Could you check a few things on this model? Use its own coordinates, in mm. Face numbers are marked on the shaded views. A direction names the side the tool comes from. Give positions to 0.01 mm unless a question says otherwise; leave off trailing zeros. Write each loop counter-clockwise with the first axis right and the second up, starting at its lowest first coordinate (ties: lowest second). Pieces come first, ordered by that corner, then holes. Notation, with made-up numbers: M 36.5,-11.75 L 59.5,-11.75 A15 cw 59.5,12.25 Z; hole C 49,-37 d3. An arc over 180 degrees is marked long. Answer as a JSON object with one key per item and string values. Group by question number.
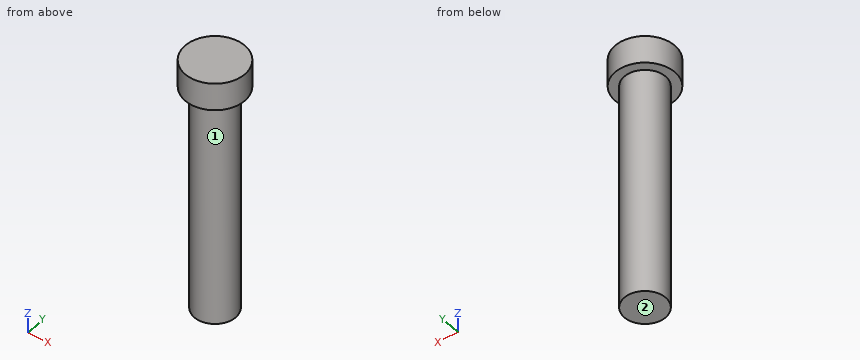
```python
from build123d import *

# Parameters (mm, degrees)
ESQUISSE1_R                    = 2.25
ESQUISSE1_R_2                  = 1.25
EXTRU_MINCE1_DEPTH             = 25
BOSS_EXTRU_1_REACH             = 14.899
ESQUISSE2_R                    = 1.25
BOSS_EXTRU_1_DIRECTION_2_REACH = 14.899
ESQUISSE3_R                    = 3.25
BOSS_EXTRU_2_DEPTH             = 3


with BuildPart() as part:
    # Esquisse1 → Extru.-Mince1 (new body)
    with BuildSketch(Plane.XY):
        Circle(ESQUISSE1_R)
        Circle(ESQUISSE1_R_2, mode=Mode.SUBTRACT)
    extrude(amount=EXTRU_MINCE1_DEPTH)

    # Boss.-Extru.1: up to this face of the body (flat: up to its plane)
    boss_extru_1_end = Plane(part.part.faces().sort_by_distance((-2.18636039, 0, 0))[0])
    # Esquisse2 → Boss.-Extru.1 (add, up to the picked face)
    with BuildSketch(Plane(origin=(0, 0, 12.5), x_dir=(-1, 0, 0), z_dir=(0, 0, -1)), mode=Mode.PRIVATE) as boss_extru_1_sk1:
        Circle(ESQUISSE2_R)
    boss_extru_1_tool1 = split(extrude(boss_extru_1_sk1.sketch, amount=BOSS_EXTRU_1_REACH, mode=Mode.PRIVATE), bisect_by=boss_extru_1_end, keep=Keep.BOTH, mode=Mode.PRIVATE)
    add(boss_extru_1_tool1.solids().sort_by(Axis((0, 0, 12.5), (0, 0, -1)))[0])

    # Boss.-Extru.1 direction 2: up to this face of the body (flat: up to its plane)
    boss_extru_1_direction_2_end = Plane(part.part.faces().sort_by_distance((-2.18636039, 0, 25))[0])
    # Esquisse2 → Boss.-Extru.1 direction 2 (add, up to the picked face)
    with BuildSketch(Plane(origin=(0, 0, 12.5), x_dir=(-1, 0, 0), z_dir=(0, 0, -1)), mode=Mode.PRIVATE) as boss_extru_1_direction_2_sk1:
        Circle(ESQUISSE2_R)
    boss_extru_1_direction_2_tool1 = split(extrude(boss_extru_1_direction_2_sk1.sketch, amount=-BOSS_EXTRU_1_DIRECTION_2_REACH, mode=Mode.PRIVATE), bisect_by=boss_extru_1_direction_2_end, keep=Keep.BOTH, mode=Mode.PRIVATE)
    add(boss_extru_1_direction_2_tool1.solids().sort_by(Axis((0, 0, 12.5), (0, 0, 1)))[0])

    # Esquisse3 → Boss.-Extru.2 (add)
    with BuildSketch(Plane.XY.offset(25)):
        Circle(ESQUISSE3_R)
    extrude(amount=BOSS_EXTRU_2_DEPTH)


solid = part.part
```
1) For the marked faces 1 and 2, which set-ups out of +Z, -Z, +X, -X, +Y, -Y let a thin tool reach every point of the face, with its end or its side?
2) If we section it at A-A, the plane y = 0: List the corners of the cut face in (x, z) for me.
3) I'm going to push flat-ended pins straight in: pin 1 (1.5 mm diameter, centred on y = 0.5, z = 8, fed in from -X); pin 2 (2 mm diameter, centred on y = 1, z = 12, fed in from +X); pin 3 (1 mm diameter, centred on x = 2, z = 21.5, fed in from +Y). Where does each tip first touch, or does it pass through?
4) If we section it at D-D, the plane y = 3: List the corners of the cut face in (x, z) for me.
5) Please list where these lines run through material, in increasing order: line 1 along Z through (x, y) = (0, 2.5); line 2 along Y through (x, z) = (0, 5.5); line 3 along X through (y, z) = (0.75, 3.5). Write a range as from..to.
6) If we section it at C-C, the plane z = 7.25: List the corners of the cut face in (x, y) for me.
Taken from the geometry:
{
 "1": {"face 1": "-Z", "face 2": "-Z, +X, -X, +Y, -Y"},
 "2": {"outline": "M -3.25,25 L -2.25,25 L -2.25,0 L 2.25,0 L 2.25,25 L 3.25,25 L 3.25,28 L -3.25,28 Z"},
 "3": {"pin 1": "x = -2.25", "pin 2": "x = 2.25", "pin 3": "y = 1.68"},
 "4": {"outline": "M -1.25,25 L 1.25,25 L 1.25,28 L -1.25,28 Z"},
 "5": {"line 1": "25..28", "line 2": "-2.25..2.25", "line 3": "-2.12..2.12"},
 "6": {"outline": "C 0,0 d4.5"}
}
